from build123d import *

# Parameters (mm, degrees)
F1_DEPTH      = 40
F1_DEPTH_BACK = 11
F4_DEPTH      = 35
F4_DEPTH_BACK = 27.9057510197
F5_T1_DEPTH   = 14.6143927182
F5_T3_DEPTH   = 14.6250082056


# Not quite as in the source:
# - a fillet or chamfer that OpenCascade refuses, or shapes differently, is made with other operations: its cross-section is extruded or revolved along the edge and cut away or added


with BuildPart() as f1:
    # F0 (on Front) → F1 (new body, two sides)
    with BuildSketch(Plane.XZ) as f1_sk:
        with BuildLine():
            Line((-16, 15.5), (-58, 15.5))
            ThreePointArc((-58, 15.5), (-58.5026261084, 7.75), (-58, 0))
            ThreePointArc((-58, 0), (-0.000843128, 1.7124660629), (58, 0.0580978101))
            ThreePointArc((58, 0.0580978101), (58.5026261084, 7.8080978101), (58, 15.5580978101))
            Line((58, 15.5580978101), (16, 15.5580978101))
            ThreePointArc((16, 15.5580978101), (0.0011638232, 14.8880205552), (-16, 15.5))
        make_face()
    extrude(amount=F1_DEPTH)
    extrude(f1_sk.sketch, amount=-F1_DEPTH_BACK)

    # F3 (on face) → F4 (cut, two sides)
    with BuildSketch(Plane(origin=(0, -8.8661687739, -10.5662884888), x_dir=(1, 0, 0), z_dir=(0, -0.6427876097, -0.7660444431))) as f4_sk:
        with BuildLine():
            Line((38.4965417924, 21), (0, 20.9813332936))
            Line((0, 20.9813332936), (-38.534011751, 20.9813332936))
            ThreePointArc((-38.534011751, 20.9813332936), (-51.7445439017, 11.0585633209), (-61, -2.6277822851))
            Line((-61, -2.6277822851), (-61, -10.626510717))
            Line((-61, -10.626510717), (-61, -28.2158330083))
            Line((-61, -28.2158330083), (0, -28.2158330083))
            Line((0, -28.2158330083), (61, -28.2158330083))
            Line((61, -28.2158330083), (61, -12.4673116952))
            Line((61, -12.4673116952), (61, -2.6264255467))
            ThreePointArc((61, -2.6264255467), (51.7297238243, 11.0740614176), (38.4965417924, 21))
        make_face()
        with BuildLine():
            Line((61, 1.9813332936), (61, 22.9813332936))
            Line((61, 22.9813332936), (61, 52.9813332936))
            Line((61, 52.9813332936), (-61, 52.9813332936))
            Line((-61, 52.9813332936), (-61, 22.9813332936))
            Line((-61, 22.9813332936), (-61, 1.9813332936))
            ThreePointArc((-61, 1.9813332936), (-51.6354627813, 14.1946752549), (-39, 22.9813332936))
            Line((-39, 22.9813332936), (39, 22.9813332936))
            ThreePointArc((39, 22.9813332936), (51.6354627813, 14.1946752549), (61, 1.9813332936))
        make_face()
    extrude(amount=-F4_DEPTH, mode=Mode.SUBTRACT)
    extrude(f4_sk.sketch, amount=F4_DEPTH_BACK, mode=Mode.SUBTRACT)

    # F5: fillet of radius 2 on 2 edges, made by hand

    # F5_s2 → F5_t1 (cut)
    with BuildSketch(Plane.XZ.offset(-0.9773730981)):
        with BuildLine():
            ThreePointArc((56.1159001591, 0.164829526), (57.5290135561, 0.6434770054), (58.2176321612, 1.9670318018))
            ThreePointArc((58.2176321612, 1.9670318018), (58.1164574753, 1.0116936322), (58, 0.0580978101))
            ThreePointArc((58, 0.0580978101), (57.0579752565, 0.1119081086), (56.1159001591, 0.164829526))
        make_face()
    extrude(amount=F5_T1_DEPTH, mode=Mode.SUBTRACT)

    # F5_s4 → F5_t3 (cut)
    with BuildSketch(Plane.XZ.offset(-0.9343439765)):
        with BuildLine():
            ThreePointArc((-58.2178227579, 1.9108828482), (-57.5284634735, 0.5866337247), (-56.1140880268, 0.1087278139))
            ThreePointArc((-56.1140880268, 0.1087278139), (-57.0570696874, 0.0548092283), (-58, 0))
            ThreePointArc((-58, 0), (-58.1165683708, 0.9545685987), (-58.2178227579, 1.9108828482))
        make_face()
    extrude(amount=F5_T3_DEPTH, mode=Mode.SUBTRACT)


solid = f1.part
Geometry: final body of the model. Coordinates: model frame, mm. A direction names the side the tool comes from. Give positions to 0.01 mm unless a question says otherwise; leave off trailing zeros. Loops run counter-clockwise (first coordinate to the right, second up) from the corner with the lowest first, then second, coordinate; pieces in that order, holes last. Notation, with made-up numbers: M 49.25,-28.5 L 93.25,-28.5 A13 ccw 93.25,-9.5 Z; hole C 26,50 d1. An arc over 180 degrees is marked long. Put each result on its own line as item: value. Start each with the question number.
1) Cut plane A-A (x = 23). Output: boundary loops of the cut face in (y, z).
2) Cut plane B-B (x = 42). Output: boundary loops of the cut face in (y, z).
3) Contact query for flat-ended pins moving along their axis: pin 1 (13 mm diameter, centred on x = -39.5, y = -7.5, fed in from +Z); pin 2 (4 mm diameter, centred on x = -30.5, z = 7, fed in from -Y); pin 3 (1 mm diameter, centred on x = 15.5, z = 4.5, fed in from +Y); pin 4 (5 mm diameter, centred on x = 29.5, y = -11, fed in from -Z). Output: stop coordinate, or through.
4) Access query for faces 4 (the cylindrical face through (-58.494, 1.686, 8.743)), 5 (the cylindrical face through (50, -9.5, 8.6)). Directions: +Z, -Z, +X, -X, +Y, -Y. A direction counts if a zero-diameter tool reaches every point of the face in a straight line with its end or side. Return the directions, or none.
5) Pull-direction query (X, two-part tool) for faces 1 (the cylindrical face through (49.76, -13.42, 8.74)), 2 (the cylindrical face through (-49.73, -9.71, 8.74)), 3 (the flat face through (-40, -14, 15.5)); classes: pulls with the +X half, pulls with the -X half, needs draft (parallel to the pull), parting line crosses it, or undercut.
6) Ray query, line 1 along X through (y, z) = (4, 11.75); line 2 along X through (y, z) = (-19, 6.75); line 3 along Y through (x, z) = (-11, 11.25). Return the intervals inside material, ascending.
Verdict:
1. outline: M -28.78,1.46 L -26.18,1.46 L -14.35,15.56 L -16.95,15.56 Z
2. outline: M -27.21,0.85 L -24.09,0.85 L -11.75,15.56 L -14.87,15.56 Z
3. pin 1: z = 15.5
3. pin 2: y = -25.8
3. pin 3: y = -23.2
3. pin 4: through
4. face 4: -X, +Y, -Y
4. face 5: -Z, +Y
5. face 1: pulls with the +X half
5. face 2: undercut
5. face 3: needs draft
6. line 1: -58.37 to -57.02, 57.02 to 58.37
6. line 2: -45.92 to -42.18, 42.18 to 45.92
6. line 3: -20.56 to -17.95
